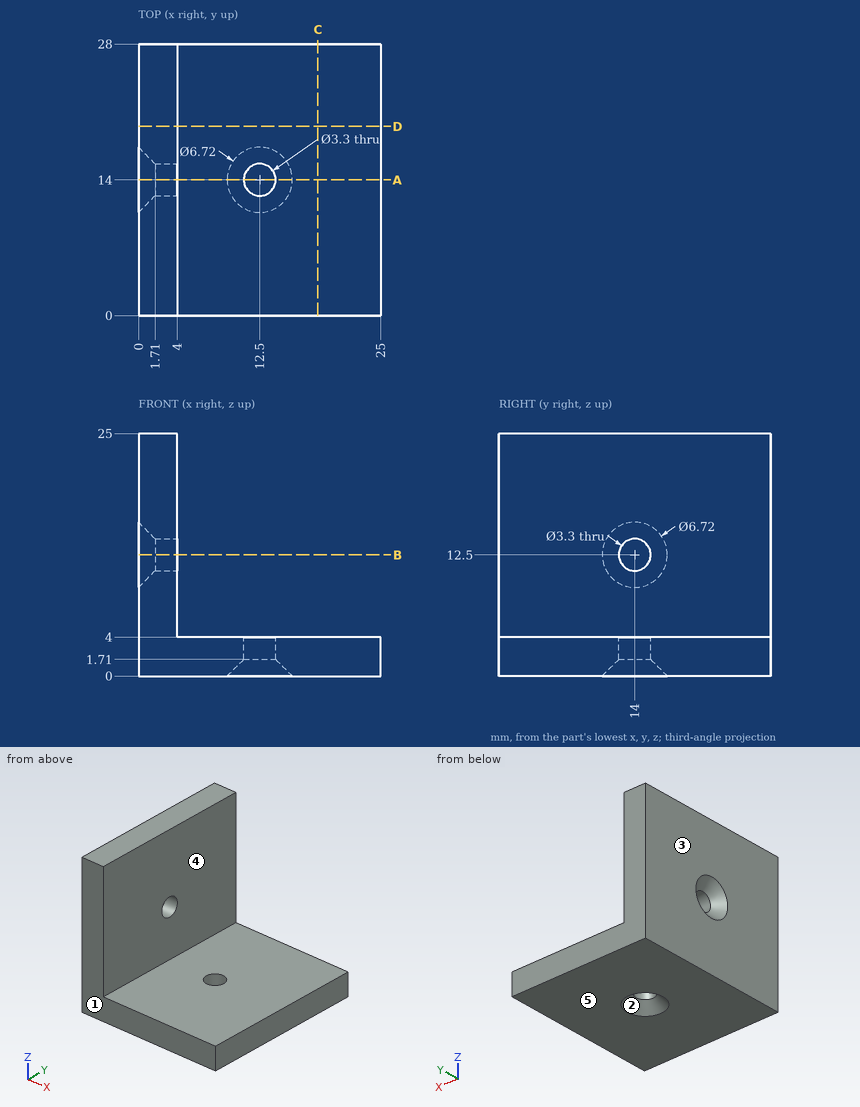
Part print with two shaded views. Sizes in mm from the minimum x, y, z corner. A direction names the side the tool comes from. Round coordinates to 2 decimals unless told otherwise and drop trailing zeros. Order: outer loops, then holes, each group sorted by start corner. A loop starts at its lowest first (then second) coordinate and runs counter-clockwise, first axis right, second up. Notation, with made-up numbers: M 56,53.5 L 78,53.5 A13 ccw 78,67.5 Z; hole C 30.5,22 d1. An arc over 180 degrees is marked long. Put each result on its own line as item: value. Start each with the question number.
1. Slice it at B-B on z = 12.5. List the corners of the cut face in (x, y), then the cut area to 3 significant figures.
2. Drill centre lines: probe 1 along Y at (x, z) = (12.5, 2.7); probe 2 along Z at (x, y) = (2.3, 14); probe 3 along X at (y, z) = (3, 21.5). Where is each one in solid material? Low to high. Write a range as [from, to].
3. Slice it at A-A on y = 14. List the corners of the cut face in (x, z).
4. Two-plate mould, pull along Y, no slides. Class the marked faces 1, 2 and 3: +Y half, -Y half, draft (parallel to the pull), parting line (faces both ways), or undercut.
5. Drop flat-ended pins along their axis: pin 1 (2 mm diameter, centred on y = 14, z = 12.5, fed in from +X); pin 2 (10 mm diameter, centred on x = 21, z = 5, fed in from +Y); pin 3 (6.5 mm diameter, centred on x = 19.5, y = 9.5, fed in from +Z); pin 4 (2 mm diameter, centred on y = 16, z = 12.5, fed in from +X). Give the stop position or say it passes through.
6. Slice it at C-C on x = 18.5. List the corners of the cut face in (y, z), then the cut area to 3 significant figures.
7. Tool access for the marked faces 4 and 5: list every direction of +Z, -Z, +X, -X, +Y, -Y with a clear straight run to the whole face (end or side of a thin tool).
8. Slice it at D-D on y = 19.5. List the corners of the cut face in (x, z), then the cut area to 3 significant figures.
Findings:
1. outline: M 0,0 L 4,0 L 4,12.35 L 1.71,12.35 L 0,10.64 Z; M 0,17.36 L 1.71,15.65 L 4,15.65 L 4,28 L 0,28 Z
1. area: 95.9 mm2
2. probe 1: [0, 12.35], [15.65, 28]
2. probe 2: [0, 10.85], [14.15, 25]
2. probe 3: [0, 4]
3. outline: M 0,0 L 9.14,0 L 10.85,1.71 L 10.85,4 L 4,4 L 4,10.85 L 1.71,10.85 L 0,9.14 Z; M 0,15.86 L 1.71,14.15 L 4,14.15 L 4,25 L 0,25 Z; M 14.15,1.71 L 15.86,0 L 25,0 L 25,4 L 14.15,4 Z
4. face 1: -Y half
4. face 2: undercut
4. face 3: draft
5. pin 1: through
5. pin 2: y = 28
5. pin 3: z = 4
5. pin 4: x = 4
6. outline: M 0,0 L 28,0 L 28,4 L 0,4 Z
6. area: 112 mm2
7. face 4: +Z, +X, +Y, -Y
7. face 5: -Z, +X, -X, +Y, -Y
8. outline: M 0,0 L 25,0 L 25,4 L 4,4 L 4,25 L 0,25 Z
8. area: 184 mm2
